from build123d import *

# Parameters (mm, degrees)
SKETCH1_R               = 4.25
BOSS_EXTRUDE1_DEPTH     = 55
SKETCH4_R               = 3
BOSS_EXTRUDE3_DEPTH     = 5
CUT_EXTRUDE2_DEPTH      = 10
CUT_EXTRUDE2_DEPTH_BACK = 10
SKETCH5_W               = 0.75
SKETCH5_H               = 7
SKETCH3_R               = 4
BOSS_EXTRUDE2_DEPTH     = 8
SKETCH6_W               = 0.8
SKETCH6_H               = 3


with BuildPart() as part:
    # Sketch1 → Boss-Extrude1 (new body)
    with BuildSketch(Plane(origin=(0, 0, 0), x_dir=(1, 0, 0), z_dir=(0, 1, 0))):
        with Locations(Location((0, 0, 0), (0, 0, 270))):
            Circle(SKETCH1_R)
    extrude(amount=BOSS_EXTRUDE1_DEPTH)

    # Sketch4 → Boss-Extrude3 (add)
    with BuildSketch(Plane(origin=(0, 55, 0), x_dir=(1, 0, 0), z_dir=(0, 1, 0))):
        with Locations(Location((0, 0, 0), (0, 0, 270))):
            Circle(SKETCH4_R)
    extrude(amount=BOSS_EXTRUDE3_DEPTH)

    # Sketch5 → Cut-Extrude2 (cut, two sides: drawn at the far end of the back side and taken through both)
    with BuildSketch(Plane.XY.offset(-CUT_EXTRUDE2_DEPTH_BACK)):
        with Locations((-3.875, 20.5)):
            Rectangle(SKETCH5_W, SKETCH5_H)
        with Locations((3.875, 20.5)):
            Rectangle(SKETCH5_W, SKETCH5_H)
    extrude(amount=CUT_EXTRUDE2_DEPTH + CUT_EXTRUDE2_DEPTH_BACK, mode=Mode.SUBTRACT)

    # Sketch3 → Boss-Extrude2 (add)
    with BuildSketch(Plane(origin=(0, 0, 0), x_dir=(1, 0, 0), z_dir=(0, 1, 0))):
        with Locations(Location((0, 0, 0), (0, 0, 270))):
            Circle(SKETCH3_R)
    extrude(amount=-BOSS_EXTRUDE2_DEPTH)

    # Sketch6 → Cut-Revolve1 (revolve, cut)
    with BuildSketch(Plane(origin=(0, 0, 0), x_dir=(0, 0, -1), z_dir=(1, 0, 0)), mode=Mode.PRIVATE) as cut_revolve1_sk:
        with Locations((3.6, -1.5)):
            Rectangle(SKETCH6_W, SKETCH6_H)
    revolve(cut_revolve1_sk.sketch.rotate(Axis((0, 55, 0), (0, -1, 0)), 180), axis=Axis((0, 55, 0), (0, -1, 0)), mode=Mode.SUBTRACT)


solid = part.part
CAD build for the part. Positions are in the model's coordinates, mm. A direction names the side the tool comes from. Coordinates: 2 decimals unless noted, no trailing zeros. Write each loop counter-clockwise with the first axis right and the second up, starting at its lowest first coordinate (ties: lowest second). Pieces come first, ordered by that corner, then holes. Notation, with made-up numbers: M -5.5,43.5 L 5.5,43.5 A9 ccw 5.5,53.5 Z; hole C 22,-14.75 d7. An arc over 180 degrees is marked long. Return JSON: item names as keys, results as strings.
Item 1: Which spindle directions (+Z, -Z, +X, -X, +Y, -Y) get a long thin tool onto all of the face, cutting with end or side? Do faces 5 (the cylindrical face through (0.187, 27.115, -4.246)), 6 (the flat face through (-3.5, 20, 0)), 7 (the cylindrical face through (0.9, 57.46, 2.86)), 8 (the flat face through (3.5, 20, 0)), 9 (the flat face through (-3, -3, 2)). Say none if no direction does.
Findings below:
{"face 5": "+Y, -Y", "face 6": "+Z, -Z, -X", "face 7": "+Y", "face 8": "+Z, -Z, +X", "face 9": "none"}
Item 2: Probe line 1 (Y direction, x = 3.75, z = -0.5); line 2 (Y direction, x = 3, z = -1.75); line 3 (X direction, y = 39, z = 0.25). List the from-to ranges inside material, lowest first. Write a range as from..to.
Findings below:
{"line 1": "y = -8..-3, 0..17, 24..55", "line 2": "y = -8..-3, 0..55", "line 3": "x = -4.24..4.24"}
Item 3: Slice it at D-D, the plane y = 56. Write the cut outline in (x, z).
Findings below:
{"outline": "C 0,0 d6"}
Item 4: Drop flat-ended pins along their axis: pin 1 Ø1 at (y, z) = (7, 2.5) entering from +X; pin 2 Ø0.6 at (x, z) = (-4, 1) entering from -Y; pin 3 Ø2.5 at (y, z) = (20.5, -1) entering from +X. Give the stop position or say it passes through.
Findings below:
{"pin 1": "stops at x = 3.75", "pin 2": "stops at y = -8", "pin 3": "stops at x = 3.5"}
Item 5: Slice it at A-A, the plane x = 0. Write the cut outline in (y, z), and give its area (3 significant figures).
Findings below:
{"outline": "M -8,-4 L -3,-4 L -3,-3.2 L 0,-3.2 L 0,-4.25 L 55,-4.25 L 55,-3 L 60,-3 L 60,3 L 55,3 L 55,4.25 L 0,4.25 L 0,3.2 L -3,3.2 L -3,4 L -8,4 Z", "area": "557 mm2"}
Item 6: Slice it at C-C, the plane y = 32.5. Write the cut outline in (x, z).
Findings below:
{"outline": "C 0,0 d8.5"}
Item 7: Two-plate mould, pull along Y, no slides. Class faces 1 (the flat face through (0, 60, 0)), 2 (the cylindrical face through (-3.905, -5.465, -0.867)), 3 (the flat face through (0, -8, 0)), 4 (the cylindrical face through (-0.961, -1.479, 3.052)): +Y half, -Y half, draft (parallel to the pull), parting line (faces both ways), or undercut.
Findings below:
{"face 1": "+Y half", "face 2": "draft", "face 3": "-Y half", "face 4": "undercut"}
Item 8: Slice it at B-B, the plane z = 0. Write the cut outline in (x, y).
Findings below:
{"outline": "M -4.25,0 L -3.2,0 L -3.2,-3 L -4,-3 L -4,-8 L 4,-8 L 4,-3 L 3.2,-3 L 3.2,0 L 4.25,0 L 4.25,17 L 3.5,17 L 3.5,24 L 4.25,24 L 4.25,55 L 3,55 L 3,60 L -3,60 L -3,55 L -4.25,55 L -4.25,24 L -3.5,24 L -3.5,17 L -4.25,17 Z"}
